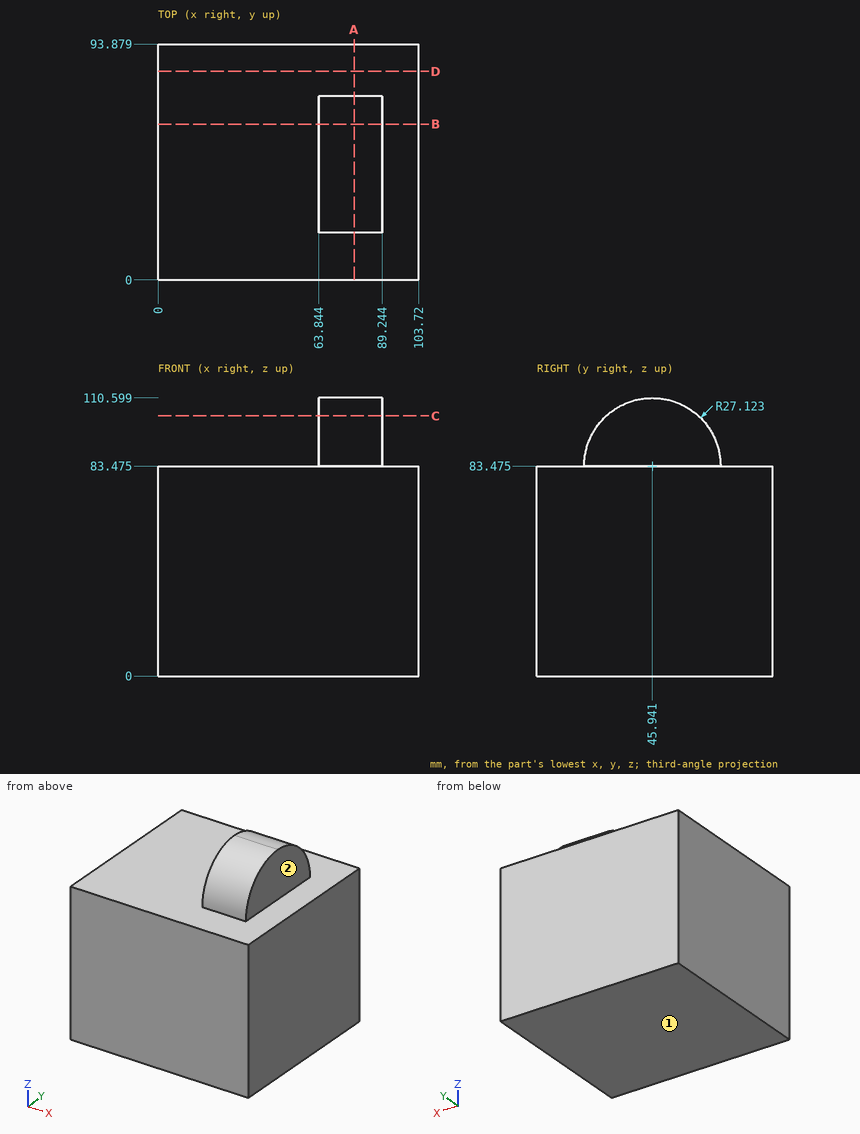
Job drawing, mm, ordinate dimensions from the low corner. One solid piece. A direction names the side the tool comes from. Round coordinates to 2 decimals unless told otherwise and drop trailing zeros. Write each loop counter-clockwise with the first axis right and the second up, starting at its lowest first coordinate (ties: lowest second). Pieces come first, ordered by that corner, then holes. Notation, with made-up numbers: (31.5, 41) -> (90.5, 41) arc R33 ccw to (90.5, 79) -> close; hole circle Ø4 at (87, -12). An arc over 180 degrees is marked (long way). Answer as CSV lines item,"result".
1. Tool access for the marked faces 1 and 2: list every direction of +Z, -Z, +X, -X, +Y, -Y with a clear straight run to the whole face (end or side of a thin tool).
Resolved:
face 1,"-Z, +X, -X, +Y, -Y"
face 2,"+Z, +X, +Y, -Y"
2. Slice it at D-D, the plane y = 83. List the corners of the cut face in (x, z) (1 decimal).
Resolved:
outline,"(0, 0) -> (103.7, 0) -> (103.7, 83.5) -> (0, 83.5) -> close"
3. Drill centre lines: line 1 (Z direction, x = 4, y = 89) (1 decimal); line 2 (Z direction, x = 85.5, y = 34.5); line 3 (X direction, y = 34.5, z = 99) (1 decimal). Where is each one in solid material? Low to high.
Resolved:
line 1,"0 to 83.5"
line 2,"0 to 108.07"
line 3,"63.8 to 89.2"
4. Slice it at C-C, the plane z = 103.5. List the corners of the cut face in (x, y) (1 decimal), plus the area to 3 significant figures.
Resolved:
outline,"(63.8, 27.6) -> (89.2, 27.6) -> (89.2, 64.2) -> (63.8, 64.2) -> close"
area,"929 mm²"
5. Pin check, flat tips, straight feed: pin 1 Ø12 at (x, y) = (21, 83.5) entering from +Z (1 decimal); pin 2 Ø13.5 at (y, z) = (43.5, 101) entering from +X; pin 3 Ø8 at (y, z) = (51.5, 93) entering from -X. Stop position of each tip, or through.
Resolved:
pin 1,"z = 83.5"
pin 2,"x = 89.24"
pin 3,"x = 63.84"
6. Slice it at B-B, the plane y = 62. List the corners of the cut face in (x, z) (1 decimal), plus the area to 3 significant figures.
Resolved:
outline,"(0, 0) -> (103.7, 0) -> (103.7, 83.5) -> (89.2, 83.5) -> (89.2, 105.3) -> (63.8, 105.3) -> (63.8, 83.5) -> (0, 83.5) -> close"
area,"9,210 mm²"
7. Slice it at A-A, the plane x = 78. List the corners of the cut face in (y, z) (1 decimal).
Resolved:
outline,"(0, 0) -> (93.9, 0) -> (93.9, 83.5) -> (73.1, 83.5) arc R27.1 ccw to (18.8, 83.5) -> (0, 83.5) -> close"
